Build history of the part. All positions in model axes, mm. Face numbers are marked on the shaded views. Round coordinates to 2 decimals unless told otherwise and drop trailing zeros. Order: outer loops, then holes, each group sorted by start corner. A loop starts at its lowest first (then second) coordinate and runs counter-clockwise, first axis right, second up. Notation, with made-up numbers: (86.5, 49.5) -> (97.5, 49.5) arc R33 ccw to (97.5, 84.5) -> close; hole circle Ø9 at (89, -27.5). An arc over 180 degrees is marked (long way). Answer as a JSON object with one key per item and string values.
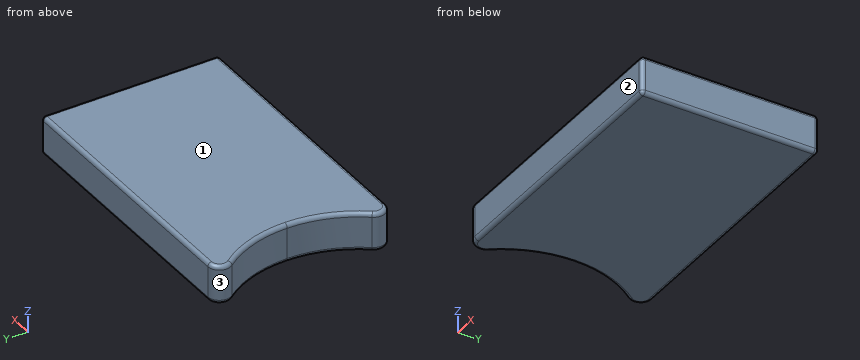
from build123d import *

# Parameters (mm, degrees)
F1_DEPTH = 12.7
F2_R     = 3.81
F3_R     = 1.27


with BuildPart() as f1:
    # F0 (on Top) → F1 (new body)
    with BuildSketch(Plane.XY):
        with BuildLine():
            Line((79.179575, 29.36875), (-18.46932, 29.36875))
            ThreePointArc((-18.46932, 29.36875), (-8.27059, 16.230849), (-4.640425, 0))
            ThreePointArc((-4.640425, 0), (-8.27059, -16.230849), (-18.46932, -29.36875))
            Line((-18.46932, -29.36875), (79.179575, -29.36875))
            Line((79.179575, -29.36875), (79.179575, 29.36875))
        make_face()
    extrude(amount=F1_DEPTH)

    # F2
    f2_edges = [f1.edges().sort_by_distance(p)[0] for p in [
        (-18.46932, 29.36875, 6.35),
        (-18.46932, -29.36875, 6.35),
    ]]
    fillet(f2_edges, radius=F2_R)

    # F3
    f3_edges = [f1.edges().sort_by_distance(p)[0] for p in [
        (34.82679, -29.36875, 12.7),
        (-12.944234, -27.241527, 12.7),
        (79.179575, 0, 12.7),
        (-4.640425, 0, 12.7),
        (34.82679, 29.36875, 12.7),
        (-12.944234, 27.241527, 12.7),
        (34.82679, -29.36875, 0),
        (-12.944234, -27.241527, 0),
        (79.179575, 0, 0),
        (-4.640425, 0, 0),
        (34.82679, 29.36875, 0),
        (-12.944234, 27.241527, 0),
        (79.179575, -29.36875, 6.35),
        (79.179575, 29.36875, 6.35),
    ]]
    fillet(f3_edges, radius=F3_R)


solid = f1.part
1) Probe L1, parallel to X at y = -27, z = 1.75; L2, parallel to X at y = 10, z = 4.5; L3, parallel to Y at x = 10, z = 1. List the from-to ranges inside material, lowest first. Write a range as from..to.
Checked values:
{"L1": "x = -13.05..79.18", "L2": "x = -5.98..79.18", "L3": "y = -29.34..29.34"}
2) Pull direction Y, two halves, no side cores. Call the marked faces 1, 2 and 3: pulls with the +Y half, pulls with the -Y half, needs draft (parallel to the pull), parting line crosses it, or undercut.
Checked values:
{"face 1": "needs draft", "face 2": "pulls with the -Y half", "face 3": "undercut"}
3) Cut at A-A, the plane z = 9. Give the cut face in (x, y), plus the area to 3 significant figures.
Checked values:
{"outline": "(-12.55, -23.24) arc R3.81 ccw to (-9.53, -29.37) -> (77.91, -29.37) arc R1.27 ccw to (79.18, -28.1) -> (79.18, 28.1) arc R1.27 ccw to (77.91, 29.37) -> (-9.53, 29.37) arc R3.81 ccw to (-12.55, 23.24) arc R38.1 cw to (-4.64, 0) arc R38.1 cw to start", "area": "5,140 mm²"}
